For this review, take the finished solid that the model builds, in its own axes (mm). A direction names the side the tool comes from. Give positions to 0.01 mm unless a question says otherwise; leave off trailing zeros. Order: outer loops, then holes, each group sorted by start corner. A loop starts at its lowest first (then second) coordinate and runs counter-clockwise, first axis right, second up.
Item 1: The part is to be moulded in two halves that separate along Z. For faces 6 (the flat face through (279.4, 6, -6)), 7 (the flat face through (276.86, 9, 0)), 8 (the cylindrical face through (137.74, -2.75, -12.4)), say which applies: released by +Z, released by -Z, zero draft, split by the parting line, or undercut.
Item 2: For probe 1 along X at (y, z) = (2, -7.75); probe 2 along Y at (x, z) = (265.5, 2.75); probe 3 along Z at (x, y) = (263.5, 5.5), list the stretches that pass through material, from the lowest coordinate up.
Item 3: For P1, Ø2, axis at x = 278.5, z = 9, coming from the -Y side; P2, Ø3, axis at x = 278.5, z = 8, coming from the +Y side; P3, Ø3, axis at x = 278, y = -9.5, coming from the +Z side, all flat-tipped, find the tip position at first contact; note any pin that passes through.
Item 4: Machinability: for faces 1 (the flat face through (0, 0, 0)), 2 (the flat face through (279.4, -6, 6)), 3 (the flat face through (260.35, 0, 0)), 4 (the flat face through (276.86, -9, 0)), 5 (the flat face through (276.86, 0, 9)), which of the approach directions +Z, -Z, +X, -X, +Y, -Y give a long, thin tool a straight path to every point of the face, cutting with its end or side? Answer none if there is none.
Item 5: Consider section A-A (z = 0). Give the boundary of the cut face in (x, y), plus the area to 3 significant figures.
Item 6: Consider section C-C (x = 219). Give the boundary of the cut face in (y, z).
```python
from build123d import *

# Parameters (mm, degrees)
F0_R     = 12.7
F1_DEPTH = 279.4
F2_R     = 6.35
F3_DEPTH = 2.54
F4_DEPTH = 19.05
F5_W     = 18.163441
F5_H     = 5.08
F5_W_2   = 5.08
F5_H_2   = 19.159987
F5_W_3   = 24.760097
F5_H_3   = 22.090506
F6_DEPTH = 2.54


with BuildPart() as f1:
    # F0 (on Right) → F1 (new body)
    with BuildSketch(Plane.YZ):
        Circle(F0_R)
    extrude(amount=F1_DEPTH)

    # F2 (on face) → F3 (cut)
    with BuildSketch(Plane.YZ.offset(279.4)):
        Circle(F2_R)
    extrude(amount=-F3_DEPTH, mode=Mode.SUBTRACT)

    # F2 (on face) → F4 (cut)
    with BuildSketch(Plane.YZ.offset(279.4)):
        Circle(F2_R)
    extrude(amount=-F4_DEPTH, mode=Mode.SUBTRACT)

    # F5 (on face) → F6 (cut)
    with BuildSketch(Plane.YZ.offset(279.4)):
        with Locations((-11.62172, 0)):
            Rectangle(F5_W, F5_H)
        with Locations((0, 12.119993)):
            Rectangle(F5_W_2, F5_H_2)
        with Locations((14.920048, 0)):
            Rectangle(F5_W_3, F5_H)
        with Locations((0, -13.585253)):
            Rectangle(F5_W_2, F5_H_3)
    extrude(amount=-F6_DEPTH, mode=Mode.SUBTRACT)


solid = f1.part
```
Resolved:
1. face 6: zero draft
1. face 7: undercut
1. face 8: split by the parting line
2. probe 1: x = 0 to 276.86
2. probe 2: y = -12.4 to -5.72, 5.72 to 12.4
2. probe 3: z = -11.45 to -3.17, 3.17 to 11.45
3. P1: stops at y = -9.86
3. P2: stops at y = 10.91
3. P3: stops at z = 9.86
4. face 1: +Z, -Z, -X, +Y, -Y
4. face 2: +Z, -Z, +X, +Y, -Y
4. face 3: +X
4. face 4: +X, +Y, -Y
4. face 5: +Z, -Z, +X
5. outline: (0, -12.7) - (276.86, -12.7) - (276.86, -6.35) - (260.35, -6.35) - (260.35, 6.35) - (276.86, 6.35) - (276.86, 12.7) - (0, 12.7) - close
5. area: 6,820 mm2
6. outline: circle Ø25.4 at (0, 0)
